from build123d import *

# Parameters (mm, degrees)
SKETCH1_R           = 1.495
SKETCH1_R_2         = 36.25
BOSS_EXTRUDE1_DEPTH = 3
SKETCH1_3_R         = 1.495
CUT_EXTRUDE2_DEPTH  = 3
SKETCH1_4_R         = 1.495
CUT_EXTRUDE3_DEPTH  = 3
SKETCH1_6_R         = 9.688899653
BOSS_EXTRUDE2_DEPTH = 40
BOSS_EXTRUDE3_START = -40
SKETCH1_7_R         = 9.688899653
SKETCH1_7_R_2       = 1.495
BOSS_EXTRUDE3_DEPTH = 40
BOSS_EXTRUDE4_START = 3
BOSS_EXTRUDE4_DEPTH = 3
SKETCH1_8_R         = 36.25
BOSS_EXTRUDE5_DEPTH = 8
BOSS_EXTRUDE6_DEPTH = 3
SKETCH4_R           = 1.495
CUT_EXTRUDE4_DEPTH  = 3


with BuildPart() as part:
    # Sketch1 → Boss-Extrude1 (new body)
    with BuildSketch(Plane.XY):
        with BuildLine():
            Line((4, 0), (156, 0))
            ThreePointArc((156, 0), (158.828427125, 1.171572875), (160, 4))
            Line((160, 4), (160, 196))
            ThreePointArc((160, 196), (158.828427125, 198.828427125), (156, 200))
            Line((156, 200), (4, 200))
            ThreePointArc((4, 200), (1.171572875, 198.828427125), (0, 196))
            Line((0, 196), (0, 4))
            ThreePointArc((0, 4), (1.171572875, 1.171572875), (4, 0))
        make_face()
        with Locations((80, 190)):
            Circle(SKETCH1_R, mode=Mode.SUBTRACT)
        with Locations((80, 100)):
            Circle(SKETCH1_R_2, mode=Mode.SUBTRACT)
    extrude(amount=BOSS_EXTRUDE1_DEPTH)

    # Sketch1_3 → Cut-Extrude2 (cut)
    with BuildSketch(Plane.XY):
        with Locations((15, 15)):
            Circle(SKETCH1_3_R)
    extrude(amount=CUT_EXTRUDE2_DEPTH, mode=Mode.SUBTRACT)

    # Sketch1_4 → Cut-Extrude3 (cut)
    with BuildSketch(Plane.XY):
        with Locations(Location((145, 15, 0), (0, 0, 180))):
            Circle(SKETCH1_4_R)
    extrude(amount=CUT_EXTRUDE3_DEPTH, mode=Mode.SUBTRACT)

    # Sketch1_6 → Boss-Extrude2 (add)
    with BuildSketch(Plane.XY):
        with Locations((145, 185)):
            Circle(SKETCH1_6_R)
    extrude(amount=-BOSS_EXTRUDE2_DEPTH)

    # Sketch1_7 → Boss-Extrude3 (add)
    # profile 1 of 3: a face of its own
    with BuildSketch(Plane.XY.offset(BOSS_EXTRUDE3_START)):
        with Locations((145, 15)):
            Circle(SKETCH1_7_R)
        with Locations(Location((145, 15, 0), (0, 0, 180))):
            Circle(SKETCH1_7_R_2, mode=Mode.SUBTRACT)
    # profile 2 of 3: a face of its own
    with BuildSketch(Plane.XY.offset(BOSS_EXTRUDE3_START)):
        with Locations((15, 15)):
            Circle(SKETCH1_7_R)
        with Locations((15, 15)):
            Circle(SKETCH1_7_R_2, mode=Mode.SUBTRACT)
    # profile 3 of 3: a face of its own
    with BuildSketch(Plane.XY.offset(BOSS_EXTRUDE3_START)):
        with Locations((15, 185)):
            Circle(SKETCH1_7_R)
    extrude(amount=BOSS_EXTRUDE3_DEPTH)

    # Sketch2 → Boss-Extrude4 (add)
    with BuildSketch(Plane(origin=(0, 0, -40), x_dir=(-1, 0, 0), z_dir=(0, 0, -1)).offset(BOSS_EXTRUDE4_START)):
        with BuildLine():
            Line((-156, 200), (-4, 200))
            ThreePointArc((-4, 200), (-1.171572875, 198.828427125), (0, 196))
            Line((0, 196), (0, 4))
            ThreePointArc((0, 4), (-1.171572875, 1.171572875), (-4, 0))
            Line((-4, 0), (-156, 0))
            ThreePointArc((-156, 0), (-158.828427125, 1.171572875), (-160, 4))
            Line((-160, 4), (-160, 196))
            ThreePointArc((-160, 196), (-158.828427125, 198.828427125), (-156, 200))
        make_face()
    extrude(amount=-BOSS_EXTRUDE4_DEPTH)

    # Sketch1_8 → Boss-Extrude5 (add)
    with BuildSketch(Plane.XY):
        with Locations((80, 100)):
            Circle(SKETCH1_8_R)
    extrude(amount=BOSS_EXTRUDE5_DEPTH)

    # Sketch3 → Boss-Extrude6 (add)
    with BuildSketch(Plane.XY.offset(3)):
        with BuildLine():
            Line((0, 68.573310073), (0, 196))
            ThreePointArc((0, 196), (1.171572875, 198.828427125), (4, 200))
            Line((4, 200), (156, 200))
            ThreePointArc((156, 200), (158.828427125, 198.828427125), (160, 196))
            Line((160, 196), (160, 68.573310073))
            Line((160, 68.573310073), (156, 68.573310073))
            Line((156, 68.573310073), (156, 192))
            ThreePointArc((156, 192), (154.828427125, 194.828427125), (152, 196))
            Line((152, 196), (8, 196))
            ThreePointArc((8, 196), (5.171572875, 194.828427125), (4, 192))
            Line((4, 192), (4, 68.573310073))
            Line((4, 68.573310073), (0, 68.573310073))
        make_face()
    extrude(amount=BOSS_EXTRUDE6_DEPTH)

    # Sketch4 → Cut-Extrude4 (cut)
    with BuildSketch(Plane.XY.offset(-40)):
        with Locations((15, 27.247777485)):
            Circle(SKETCH4_R)
        with Locations(Location((145, 27.247777485, 0), (0, 0, 180))):
            Circle(SKETCH4_R)
        with Locations((145, 172.752222515)):
            Circle(SKETCH4_R)
        with Locations(Location((15, 172.752222515, 0), (0, 0, 180))):
            Circle(SKETCH4_R)
        with Locations((15, 129.079723254)):
            Circle(SKETCH4_R)
        with Locations((15, 70.716662913)):
            Circle(SKETCH4_R)
        with Locations(Location((145, 70.716662913, 0), (0, 0, 180))):
            Circle(SKETCH4_R)
        with Locations(Location((145, 129.079723254, 0), (0, 0, 180))):
            Circle(SKETCH4_R)
    extrude(amount=-CUT_EXTRUDE4_DEPTH, mode=Mode.SUBTRACT)


solid = part.part
Verification items for the finished model (mm, model axes). A direction names the side the tool comes from. Give positions to 0.01 mm unless a question says otherwise; leave off trailing zeros. Loops run counter-clockwise (first coordinate to the right, second up) from the corner with the lowest first, then second, coordinate; pieces in that order, holes last. Notation, with made-up numbers: (-36, 50) - (-19, 50) arc R29 ccw to (-19, 89) - close; hole circle Ø1 at (4.5, -39). An arc over 180 degrees is marked (long way). Write item = value, one per line. Start each with the question number.
Q1. Thickness scan on line 1 (Y direction, x = 15, z = -42.25); line 2 (Y direction, x = 15, z = -23) (3 decimals); line 3 (Z direction, x = 113, y = 122). Record the ranges inside material, lowest first.
Q2. Tool access check on faces 1 (the face through (80, 198, 6)), 2 (the face through (114.576, 110.889, 5.465)), 3 (the face through (154.859, 194.797, 4.479)), 4 (the face through (79, 101, -40)). Record the directions out of +Z, -Z, +X, -X, +Y, -Y that give a thin tool (end or side, any length) a straight path to the whole face; none if there is none.
Q3. Mould release check, pull along X, two halves, no side actions. Record for faces 5 (the face through (137.86, 21.55, -20.28)), 6 (the face through (160, 123, 3)), 7 (the face through (0, 120, 3)): released by +X, released by -X, zero draft, split by the parting line, or undercut.
Q4. Cross-section at B-B, the plane x = 125.5. Enter the section's corners in (y, z), and give its area (3 significant figures).
Q5. Depth check by flat-ended pin: P1, Ø3.5, axis at x = 145, y = 15, coming from the +Z side; P2, Ø1.8, axis at x = 15, y = 70.72, coming from the -Z side; P3, Ø3.5, axis at x = 91.5, z = 5, coming from the -Y side; P4, Ø3.5, axis at x = 145, y = 129.08, coming from the -Z side. Enter the tip coordinate at first touch or a pass-through.
Q6. Cross-section at C-C, the plane z = -4. Enter the section's corners in (x, y) (3 decimals), and give its area (3 significant figures).
Q7. Cross-section at A-A, the plane y = 100. Enter the section's corners in (x, z).
Q8. Cross-section at D-D, the plane y = 147. Enter the section's corners in (x, z), and give its area (3 significant figures).
Answer key:
q1.line_1 = 0 to 25.75, 28.74 to 69.22, 72.21 to 127.58, 130.57 to 171.26, 174.25 to 200
q1.line_2 = 5.311 to 13.505, 16.495 to 24.689, 175.311 to 194.689
q1.line_3 = -43 to -40, 0 to 3
q2.face_1 = +Z, +Y
q2.face_2 = +Z
q2.face_3 = +Z, -Y
q2.face_4 = none
q3.face_5 = undercut
q3.face_6 = released by +X
q3.face_7 = released by -X
q4.outline = (0, -43) - (200, -43) - (200, -40) - (0, -40) - close; (0, 0) - (200, 0) - (200, 6) - (196, 6) - (196, 3) - (0, 3) - close
q4.area = 1,210 mm^2
q5.P1 = 3
q5.P2 = 0
q5.P3 = 65.09
q5.P4 = -43
q6.outline = circle Ø19.378 at (15, 15); circle Ø19.378 at (15, 185); circle Ø19.378 at (145, 15); circle Ø19.378 at (145, 185); hole circle Ø2.99 at (15, 15); hole circle Ø2.99 at (145, 15)
q6.area = 1,170 mm^2
q7.outline = (0, -43) - (160, -43) - (160, -40) - (0, -40) - close; (0, 0) - (160, 0) - (160, 6) - (156, 6) - (156, 3) - (116.25, 3) - (116.25, 8) - (43.75, 8) - (43.75, 3) - (4, 3) - (4, 6) - (0, 6) - close
q8.outline = (0, -43) - (160, -43) - (160, -40) - (0, -40) - close; (0, 0) - (160, 0) - (160, 6) - (156, 6) - (156, 3) - (4, 3) - (4, 6) - (0, 6) - close
q8.area = 984 mm^2
